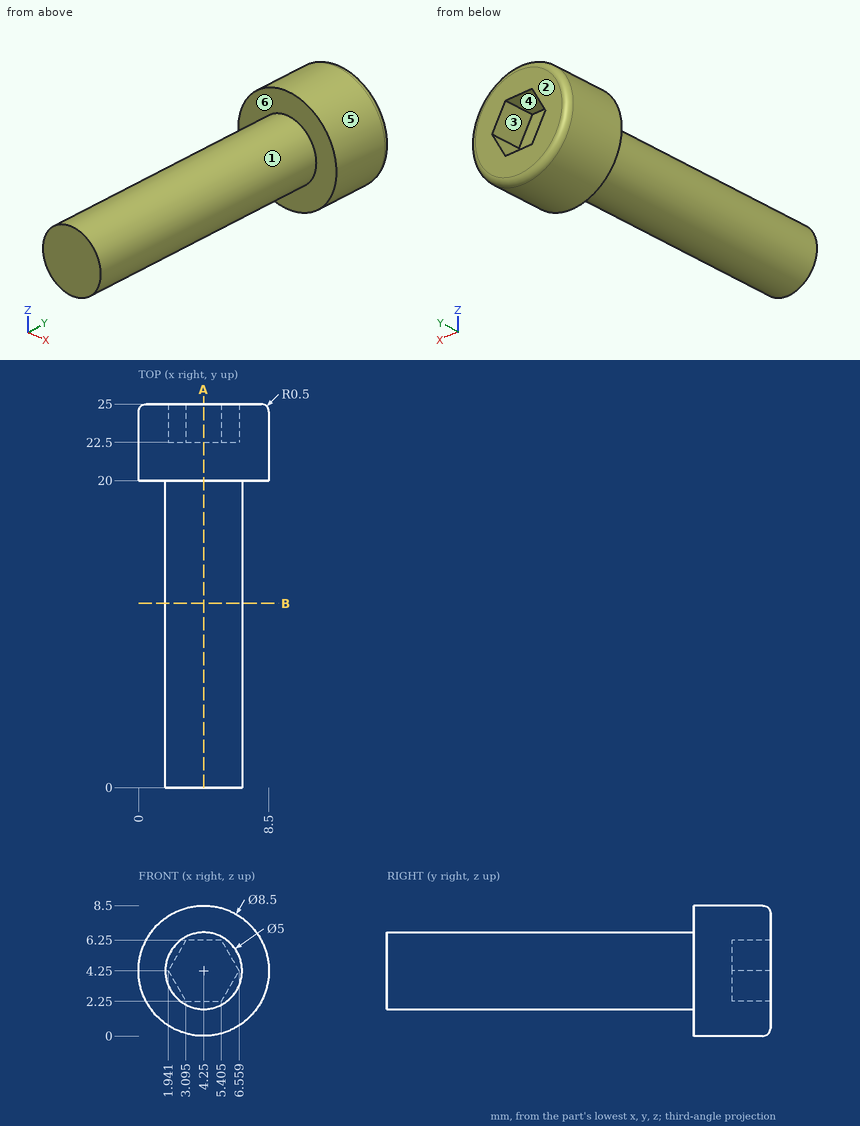
Geometry check sheet. Reference: drawing and pictorial views, mm from the part's lowest x, y, z. A direction names the side the tool comes from. Round coordinates to 2 decimals unless told otherwise and drop trailing zeros. Write each loop counter-clockwise with the first axis right and the second up, starting at its lowest first coordinate (ties: lowest second). Pieces come first, ordered by that corner, then holes.
Item 1: Section check A-A (x = 4.25). Record the boundary of the cut face in (y, z).
Determined:
outline: (0, 1.75) - (20, 1.75) - (20, 0) - (24.5, 0) arc R0.5 ccw to (25, 0.5) - (25, 2.25) - (22.5, 2.25) - (22.5, 6.25) - (25, 6.25) - (25, 8) arc R0.5 ccw to (24.5, 8.5) - (20, 8.5) - (20, 6.75) - (0, 6.75) - close
Item 2: Go/stop test with flat-tipped pins: pin 1 Ø1.5 at (x, y) = (5.5, 16.5) entering from +Z; pin 2 Ø2 at (y, z) = (18, 4.5) entering from +X. Record where each tip stops, or that it passes through.
Determined:
pin 1: stops at z = 6.7
pin 2: stops at x = 6.75
Item 3: Section check B-B (y = 12). Record the boundary of the cut face in (x, z).
Determined:
outline: circle Ø5 at (4.25, 4.25)
Item 4: Mould release check, pull along Z, two halves, no side actions. Record for the marked faces 4, 5 and 6: +Z half, -Z half, draft (parallel to the pull), parting line (faces both ways), or undercut.
Determined:
face 4: undercut
face 5: parting line
face 6: draft
Item 5: Material ranges on line 1 along Z through (x, y) = (4.25, 15.25); line 2 along X through (y, z) = (13.25, 5.75); line 3 along Y through (x, z) = (6.75, 5.25), recorded low to high.
Determined:
line 1: z = 1.75 to 6.75
line 2: x = 2.25 to 6.25
line 3: y = 20 to 25
Item 6: Access from +Z, -Z, +X, -X, +Y, -Y to the whole of each face (thin tool, end or side, straight path). Record for the marked faces 1, 2 and 3.
Determined:
face 1: -Y
face 2: +Z, -Z, +X, -X, +Y
face 3: +Y
